Check sheet for the modelled part. Datum: model origin and axes. Units: mm. Face numbers are marked on the shaded views. Round coordinates to 2 decimals unless told otherwise and drop trailing zeros. Loops run counter-clockwise (first coordinate to the right, second up) from the corner with the lowest first, then second, coordinate; pieces in that order, holes last. Notation, with made-up numbers: (72.5, -16.75) - (122.5, -16.75) arc R25 ccw to (122.5, 6.25) - close; hole circle Ø11 at (68.5, 7). An arc over 180 degrees is marked (long way). Return JSON: item names as keys, results as strings.
from build123d import *

# Parameters (mm, degrees)
SKETCH1_W               = 250
SKETCH1_H               = 40
BOSS_EXTRUDE1_DEPTH     = 40
CUT_EXTRUDE1_DEPTH      = 278.634133017
CUT_EXTRUDE1_DEPTH_BACK = 278.634133017
SKETCH2_W               = 30
SKETCH2_H               = 30
CUT_EXTRUDE2_DEPTH      = 178.338713683
CUT_EXTRUDE2_DEPTH_BACK = 178.338713683
SKETCH3_W               = 80
SKETCH3_H               = 20
CUT_EXTRUDE3_DEPTH      = 142.662654059
CUT_EXTRUDE3_DEPTH_BACK = 142.662654059
SKETCH4_W               = 80
SKETCH4_H               = 20
CUT_EXTRUDE4_DEPTH      = 178.338713683
CUT_EXTRUDE4_DEPTH_BACK = 178.338713683
SKETCH5_W               = 20
SKETCH5_H               = 20
SKETCH6_R               = 10
BOSS_EXTRUDE2_DEPTH     = 40
SKETCH7_R               = 20
BOSS_EXTRUDE3_DEPTH     = 40
CUT_EXTRUDE5_DEPTH      = 161.198094577
CUT_EXTRUDE5_DEPTH_BACK = 161.198094577
SKETCH8_R               = 10


with BuildPart() as part:
    # Sketch1 → Boss-Extrude1 (new body)
    with BuildSketch(Plane.XY):
        with Locations((4.87804878, -93.932926829)):
            Rectangle(SKETCH1_W, SKETCH1_H)
    extrude(amount=BOSS_EXTRUDE1_DEPTH)

    # Sketch2 → Cut-Extrude1 (cut, two sides: drawn at the far end of the back side and taken through both)
    with BuildSketch(Plane(origin=(129.87804878, 0, 0), x_dir=(0, 0, -1), z_dir=(1, 0, 0)).offset(-CUT_EXTRUDE1_DEPTH_BACK)):
        with Locations((-20, -93.932926829)):
            Rectangle(SKETCH2_W, SKETCH2_H)
    extrude(amount=CUT_EXTRUDE1_DEPTH + CUT_EXTRUDE1_DEPTH_BACK, mode=Mode.SUBTRACT)

    # Sketch3 → Cut-Extrude2 (cut, two sides: drawn at the far end of the back side and taken through both)
    with BuildSketch(Plane(origin=(0, 0, 0), x_dir=(-1, 0, 0), z_dir=(0, 0, -1)).offset(-CUT_EXTRUDE2_DEPTH_BACK)):
        with Locations((-59.87804878, -93.932926829)):
            Rectangle(SKETCH3_W, SKETCH3_H)
        with Locations((50.12195122, -93.932926829)):
            Rectangle(SKETCH3_W, SKETCH3_H)
    extrude(amount=CUT_EXTRUDE2_DEPTH + CUT_EXTRUDE2_DEPTH_BACK, mode=Mode.SUBTRACT)

    # Sketch4 → Cut-Extrude3 (cut, two sides: drawn at the far end of the back side and taken through both)
    with BuildSketch(Plane(origin=(0, -73.932926829, 0), x_dir=(1, 0, 0), z_dir=(0, 1, 0)).offset(-CUT_EXTRUDE3_DEPTH_BACK)):
        with Locations((59.87804878, -20)):
            Rectangle(SKETCH4_W, SKETCH4_H)
        with Locations((-50.12195122, -20)):
            Rectangle(SKETCH4_W, SKETCH4_H)
    extrude(amount=CUT_EXTRUDE3_DEPTH + CUT_EXTRUDE3_DEPTH_BACK, mode=Mode.SUBTRACT)

    # Sketch5 → Cut-Extrude4 (cut, two sides: drawn at the far end of the back side and taken through both)
    with BuildSketch(Plane.XY.offset(40).offset(-CUT_EXTRUDE4_DEPTH_BACK)):
        with Locations((-110.12195122, -93.932926829)):
            Rectangle(SKETCH5_W, SKETCH5_H)
    extrude(amount=CUT_EXTRUDE4_DEPTH + CUT_EXTRUDE4_DEPTH_BACK, mode=Mode.SUBTRACT)

    # Sketch6 → Boss-Extrude2 (add)
    with BuildSketch(Plane.XZ.offset(113.932926829)):
        with Locations(Location((-115.12195122, 20, 0), (0, 0, 240))):
            Circle(SKETCH6_R)
    extrude(amount=-BOSS_EXTRUDE2_DEPTH)

    # Sketch7 → Boss-Extrude3 (add)
    with BuildSketch(Plane.XZ.offset(113.932926829)):
        with Locations((129.87804878, 20)):
            Circle(SKETCH7_R)
    extrude(amount=-BOSS_EXTRUDE3_DEPTH)

    # Sketch8 → Cut-Extrude5 (cut, two sides: drawn at the far end of the back side and taken through both)
    with BuildSketch(Plane(origin=(0, -113.932926829, 0), x_dir=(-1, 0, 0), z_dir=(0, -1, 0)).offset(-CUT_EXTRUDE5_DEPTH_BACK)):
        with Locations(Location((-129.87804878, -20, 0), (0, 0, 90))):
            Circle(SKETCH8_R)
    extrude(amount=CUT_EXTRUDE5_DEPTH + CUT_EXTRUDE5_DEPTH_BACK, mode=Mode.SUBTRACT)


solid = part.part
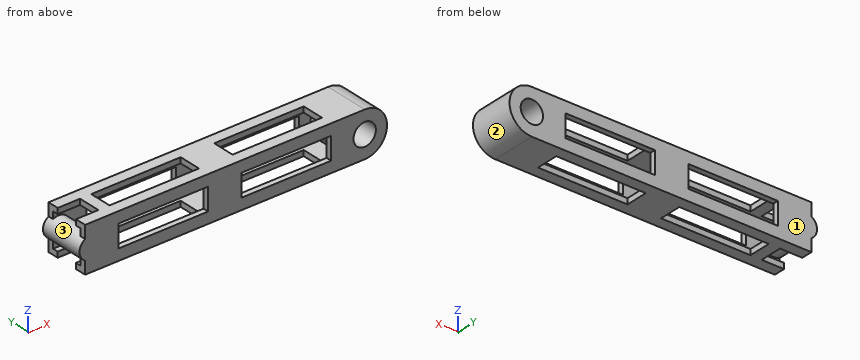
Q1. Scan lines: probe 1 along Z at (x, y) = (16.5, -104); probe 2 along Y at (x, z) = (-56, 33); probe 3 along X at (y, z) = (-105, 26). Record each from-to range of solid material in increasing order. Write a range as [from, to].
Answer key:
{"probe 1": "z = [0, 5], [35, 40]", "probe 2": "y = [-113.93, -108.93], [-78.93, -73.93]", "probe 3": "x = [-123.12, -107.12], [110.8, 121.88], [137.88, 148.96]"}
Q2. Depth check by flat-ended pin: P1, Ø11, axis at y = -79, z = 33, coming from the -X side; P2, Ø5, axis at y = -81.5, z = 30.5, coming from the -X side; P3, Ø4, axis at y = -94, z = 3.5, coming from the -X side. Enter the tip coordinate at first touch or a pass-through.
Answer key:
{"P1": "stops at x = -121.74", "P2": "stops at x = -121.12", "P3": "stops at x = -100.12"}
Q3. Sectioned sample at A-A (y = -89). Enter the section's corners in (x, z).
Answer key:
{"outline": "circle Ø20 at (-115.12, 20); (-100.12, 0) - (-90.12, 0) - (-90.12, 5) - (-100.12, 5) - close; (-100.12, 35) - (-90.12, 35) - (-90.12, 40) - (-100.12, 40) - close; (-10.12, 0) - (19.88, 0) - (19.88, 5) - (-10.12, 5) - close; (-10.12, 35) - (19.88, 35) - (19.88, 40) - (-10.12, 40) - close; (99.88, 0) - (129.88, 0) arc R20 ccw to (129.88, 40) - (99.88, 40) - (99.88, 35) - (116.65, 35) arc R20 ccw to (116.65, 5) - (99.88, 5) - close; hole circle Ø20 at (129.88, 20)"}
Q4. Sectioned sample at B-B (z = 20). Enter the section's corners in (x, y), plus the area to 3 significant figures.
Answer key:
{"outline": "(-125.12, -113.93) - (-90.12, -113.93) - (-90.12, -108.93) - (-105.12, -108.93) - (-105.12, -78.93) - (-90.12, -78.93) - (-90.12, -73.93) - (-125.12, -73.93) - close; (-10.12, -113.93) - (19.88, -113.93) - (19.88, -108.93) - (-10.12, -108.93) - close; (-10.12, -78.93) - (19.88, -78.93) - (19.88, -73.93) - (-10.12, -73.93) - close; (99.88, -113.93) - (119.88, -113.93) - (119.88, -73.93) - (99.88, -73.93) - (99.88, -78.93) - (109.88, -78.93) - (109.88, -108.93) - (99.88, -108.93) - close; (139.88, -113.93) - (149.88, -113.93) - (149.88, -73.93) - (139.88, -73.93) - close", "area": "2,150 mm²"}
Q5. Sectioned sample at C-C (x = 95). Enter the section's corners in (y, z), plus the area to 3 significant figures.
Answer key:
{"outline": "(-113.93, 0) - (-103.93, 0) - (-103.93, 5) - (-108.93, 5) - (-108.93, 10) - (-113.93, 10) - close; (-113.93, 30) - (-108.93, 30) - (-108.93, 35) - (-103.93, 35) - (-103.93, 40) - (-113.93, 40) - close; (-83.93, 0) - (-73.93, 0) - (-73.93, 10) - (-78.93, 10) - (-78.93, 5) - (-83.93, 5) - close; (-83.93, 35) - (-78.93, 35) - (-78.93, 30) - (-73.93, 30) - (-73.93, 40) - (-83.93, 40) - close", "area": "300 mm²"}
Q6. Draft check along Z on the marked faces 1, 2 and 3. Enter one of: released by +Z, released by -Z, zero draft, split by the parting line, or undercut.
Answer key:
{"face 1": "zero draft", "face 2": "split by the parting line", "face 3": "undercut"}
